Input: dimensioned drawing with shaded views. Units: mm. Origin: part minimum x, y, z. A direction names the side the tool comes from. Round coordinates to 2 decimals unless told otherwise and drop trailing zeros. Write each loop counter-clockwise with the first axis right and the second up, starting at its lowest first coordinate (ties: lowest second). Pieces come first, ordered by that corner, then holes. Notation, with made-up numbers: (62, 84) -> (108, 84) arc R27 cw to (108, 112) -> close; hole circle Ø11 at (48.25, 42.25). An arc over 180 degrees is marked (long way). Use one line per item in the form item = value. Start each with the question number.
1. Draft query along Z for the marked faces 3, 4, 5 and 6. Return one class per face: pulls with the +Z half, pulls with the -Z half, needs draft (parallel to the pull), parting line crosses it, or undercut.
2. Cut plane D-D, the plane x = 36. Return the cut outline in (y, z), plus the area to 3 significant figures.
3. Cut plane B-B, the plane x = 74.5. Return the cut outline in (y, z), plus the area to 3 significant figures.
4. Cut plane A-A, the plane z = 13. Return the cut outline in (x, y).
5. Line query: L1, parallel to X at y = 51, z = 28; L2, parallel to Z at x = 25, y = 28.5; L3, parallel to X at y = 32.5, z = 10.5. Output: solid intervals per line, ascending.
6. Reachability of the marked faces 1 and 2 from +Z, -Z, +X, -X, +Y, -Y: full face, straight path, thin tool, end or side. Return the list, or none.
7. Cut plane C-C, the plane y = 34. Return the cut outline in (x, z), plus the area to 3 significant figures.
8. Pin query (flat end, axial travel): pin 1 Ø24 at (x, z) = (57, 38.5) entering from +Y; pin 2 Ø1.5 at (x, z) = (45, 29) entering from +Y; pin 3 Ø12.5 at (y, z) = (23.5, 25) entering from +X. Return the tip coordinate at first contact, or that it passes through.
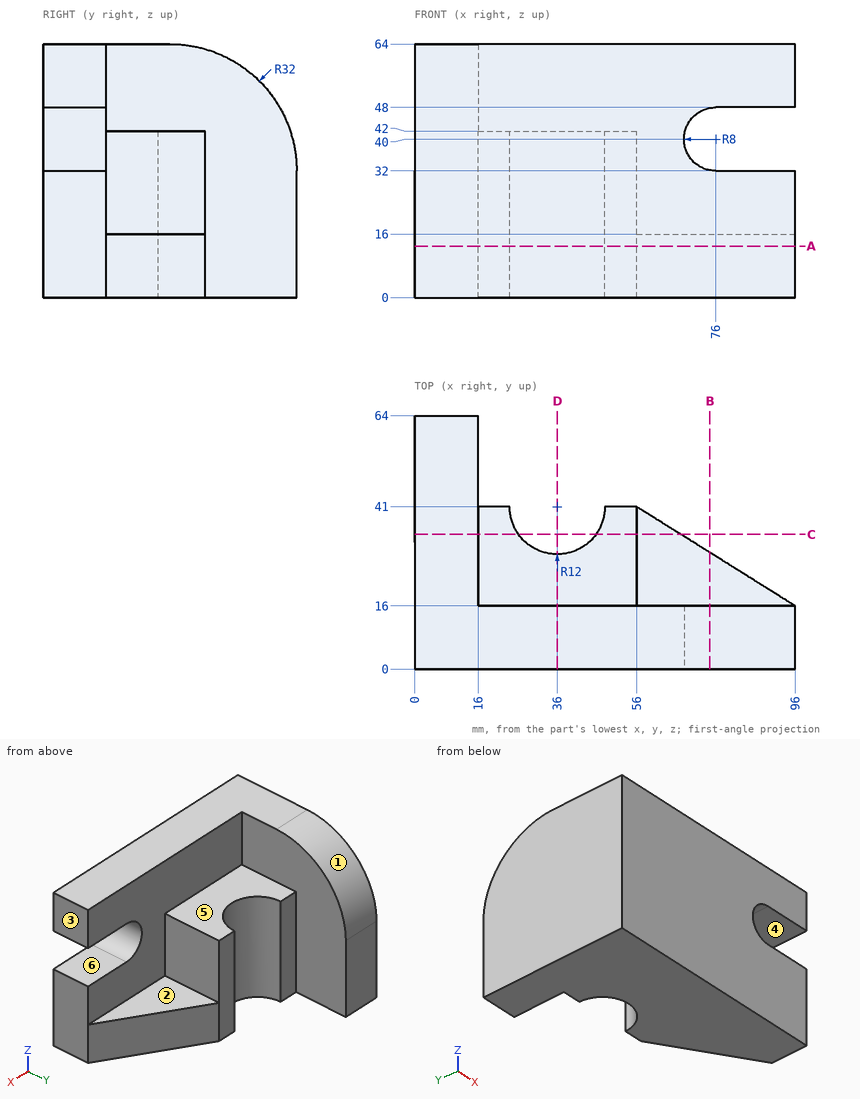
Outcome:
q1.face_3 = needs draft
q1.face_4 = undercut
q1.face_5 = pulls with the +Z half
q1.face_6 = undercut
q2.outline = (0, 0) -> (29, 0) -> (29, 42) -> (16, 42) -> (16, 64) -> (0, 64) -> close
q2.area = 1,570 mm^2
q3.outline = (0, 0) -> (29.44, 0) -> (29.44, 16) -> (16, 16) -> (16, 32.14) -> (0, 32.14) -> close; (0, 47.86) -> (16, 47.86) -> (16, 64) -> (0, 64) -> close
q3.area = 988 mm^2
q4.outline = (0, 0) -> (96, 0) -> (96, 16) -> (56, 41) -> (48, 41) arc R12 cw to (24, 41) -> (16, 41) -> (16, 64) -> (0, 64) -> close
q5.L1 = 0 to 16
q5.L2 = 0 to 42
q5.L3 = 0 to 27.53, 44.47 to 69.6
q6.face_1 = +Z, +X, -X, +Y
q6.face_2 = +Z, +X, +Y
q7.outline = (0, 0) -> (26.25, 0) -> (26.25, 42) -> (16, 42) -> (16, 63.94) -> (0, 63.94) -> close; (45.75, 0) -> (67.2, 0) -> (67.2, 16) -> (56, 16) -> (56, 42) -> (45.75, 42) -> close
q7.area = 2,060 mm^2
q8.pin_1 = 41
q8.pin_2 = 34
q8.pin_3 = 56
